from build123d import *

# Parameters (mm, degrees)
PAD_DEPTH    = 7.5
SKETCH001_R  = 1.5
POCKET_DEPTH = 4
SKETCH004_R  = 1.5
PAD001_DEPTH = 5


with BuildPart() as part:
    # Sketch → Pad (new body, symmetric)
    with BuildSketch(Plane.XY):
        Polygon((2.6, 1.501111), (0, 3.002221), (-2.6, 1.501111), (-2.6, -1.501111), (0, -3.002221), (2.6, -1.501111), align=None)
    extrude(amount=PAD_DEPTH, both=True)

    # Sketch001 (on Face8 of Pad) → Pocket (cut)
    with BuildSketch(Plane.XY.offset(7.5)):
        Circle(SKETCH001_R)
    extrude(amount=-POCKET_DEPTH, mode=Mode.SUBTRACT)

    # Sketch004 (on Face4 of Pocket) → Pad001 (join)
    with BuildSketch(Plane(origin=(0, 0, -7.5), x_dir=(1, 0, 0), z_dir=(0, 0, -1))):
        Circle(SKETCH004_R)
    extrude(amount=PAD001_DEPTH)

    # Sketch005 → Groove (revolve, cut)
    with BuildSketch(Plane.YZ):
        Polygon((2, 8), (6, 8), (6, -8), (2, -8), (5, -5), (5, 5), align=None)
    revolve(axis=Axis((0, 0, 0), (0, 0, 1)), mode=Mode.SUBTRACT)


solid = part.part
Geometry check sheet. Reference: the model listing, model coordinates, mm. A direction names the side the tool comes from. Give positions to 0.01 mm unless a question says otherwise; leave off trailing zeros. Write each loop counter-clockwise with the first axis right and the second up, starting at its lowest first coordinate (ties: lowest second). Pieces come first, ordered by that corner, then holes. Notation, with made-up numbers: (2, 74) - (8, 74) arc R19 cw to (8, 81) - close; hole circle Ø11 at (70, 42). An arc over 180 degrees is marked (long way). Put each result on its own line as item: value.
1. Draft check along X on faces 3 (the flat face through (-2.6, 0, 0)), 4 (the cylindrical face through (-1.5, 0.07, 5.53)), 5 (the flat face through (0, 0, 3.5)), 6 (the flat face through (2, 0, 7.5)). Enter one of: +X half, -X half, draft (parallel to the pull), parting line (faces both ways), or undercut.
Ans:
face 3: -X half
face 4: undercut
face 5: undercut
face 6: draft
2. Sectioned sample at B-B, the plane z = -0.5. Enter the section's corners in (x, y), plus the area to 3 significant figures.
Ans:
outline: (-2.6, -1.5) - (0, -3) - (2.6, -1.5) - (2.6, 1.5) - (0, 3) - (-2.6, 1.5) - close
area: 23.4 mm²
3. Sectioned sample at A-A, the plane y = 0. Enter the section's corners in (x, z), plus the area to 3 significant figures.
Ans:
outline: (-2.6, -7.4) - (-2.5, -7.5) - (-1.5, -7.5) - (-1.5, -12.5) - (1.5, -12.5) - (1.5, -7.5) - (2.5, -7.5) - (2.6, -7.4) - (2.6, 7.4) - (2.5, 7.5) - (1.5, 7.5) - (1.5, 3.5) - (-1.5, 3.5) - (-1.5, 7.5) - (-2.5, 7.5) - (-2.6, 7.4) - close
area: 81.0 mm²
4. Go/stop test with flat-tipped pins: pin 1 (1 mm diameter, centred on x = -1.5, y = 1.5, fed in from -Z); pin 2 (2 mm diameter, centred on x = -2, z = -6.5, fed in from -Y); pin 3 (1.5 mm diameter, centred on x = 0, y = 0.5, fed in from +Z). Record where each tip stops, or that it passes through.
Ans:
pin 1: stops at z = -7.5
pin 2: stops at y = -2.42
pin 3: stops at z = 3.5
5. Sectioned sample at C-C, the plane z = -11. Enter the section's corners in (x, y).
Ans:
outline: circle Ø3 at (0, 0)
6. Set-up check for faces 1 (the flat face through (1.282, -2.262, 0.104)), 2 (the flat face through (2, 0, -7.5)): record each of +Z, -Z, +X, -X, +Y, -Y from which the full face is reachable in a straight line by a thin tool's end or side.
Ans:
face 1: +Z, -Z, +X, -Y
face 2: -Z
7. Thickness scan on line 1 (Z direction, x = 1.5, y = 0.75); line 2 (Z direction, x = -0.85, y = -0.5); line 3 (Y direction, x = 0.35, z = 6.25). Record the ranges inside material, lowest first.
Ans:
line 1: z = -7.5 to 7.5
line 2: z = -12.5 to 3.5
line 3: y = -2.8 to -1.46, 1.46 to 2.8
